```python
from build123d import *

# Parameters (mm, degrees)
SKETCH1_R           = 98.425
SKETCH1_R_2         = 8.89
BOSS_EXTRUDE1_DEPTH = 3.175


with BuildPart() as part:
    # Sketch1 → Boss-Extrude1 (new body)
    with BuildSketch(Plane(origin=(0, 0, 0), x_dir=(1, 0, 0), z_dir=(0, 1, 0))):
        Circle(SKETCH1_R)
        Circle(SKETCH1_R_2, mode=Mode.SUBTRACT)
        with BuildLine():
            Line((-5.5, 22.5), (-5.5, 67.5))
            ThreePointArc((-5.5, 67.5), (0, 73), (5.5, 67.5))
            Line((5.5, 67.5), (5.5, 22.5))
            ThreePointArc((5.5, 22.5), (0, 17), (-5.5, 22.5))
        make_face(mode=Mode.SUBTRACT)
    extrude(amount=BOSS_EXTRUDE1_DEPTH)


solid = part.part
```
Geometry: final body of the model. Coordinates: model frame, mm. A direction names the side the tool comes from. Coordinates: 2 decimals unless noted, no trailing zeros. Write each loop counter-clockwise with the first axis right and the second up, starting at its lowest first coordinate (ties: lowest second). Pieces come first, ordered by that corner, then holes. Notation, with made-up numbers: M -23,-19.75 L 29,-19.75 A9 cw 29,-4.75 Z; hole C 18,42.25 d6. An arc over 180 degrees is marked long. Use CSV: the item, a comma, the result in double quotes. Start each with the question number.
1. Mould query, pull axis Z, two halves, no side actions, for faces 3 (the face through (-1.93, 1.57, 8.68)), 4 (the face through (-1, 0, 20)), 5 (the face through (93.88, 1.57, -29.56)). Classes: pulls with the +Z half, pulls with the -Z half, needs draft (parallel to the pull), parting line crosses it, or undercut.
2. First-contact query: P1, Ø1.5, axis at y = 1, z = -68, coming from the +X side; P2, Ø1.5, axis at y = 0.5, z = 78, coming from the -X side; P3, Ø1.6, axis at y = 1, z = -38.5, coming from the +X side. Flat tips, straight axial feed; report the tip coordinate or a pass-through.
3. Cut plane A-A on x = 0. Return the cut outline in (y, z) (3 decimals).
4. Cut plane D-D on z = -25.5. Return the cut outline in (x, y) (3 decimals).
5. Cut plane C-C on y = 1.9. Return the cut outline in (x, z) (3 decimals), plus the area to 3 significant figures.
6. Reachability of faces 1 (the face through (-1, 3.175, 20)), 2 (the face through (0, 2, -73)) from +Z, -Z, +X, -X, +Y, -Y: full face, straight path, thin tool, end or side. Return the list, or none.
7. Ray query, probe 1 along Z at (x, y) = (0, 0.95) (3 decimals); probe 2 along X at (y, z) = (0.9, 0) (3 decimals); probe 3 along X at (y, z) = (0.8, 2.5). Return the intervals inside material, ascending.
8. Cut plane B-B on z = 0. Return the cut outline in (x, y) (3 decimals), plus the area to 3 significant figures.
Entries:
1,face 3,"undercut"
1,face 4,"needs draft"
1,face 5,"parting line crosses it"
2,P1,"x = 71.87"
2,P2,"x = -60.99"
2,P3,"x = 90.92"
3,outline,"M 0,-98.425 L 3.175,-98.425 L 3.175,-73 L 0,-73 Z; M 0,-17 L 3.175,-17 L 3.175,-8.89 L 0,-8.89 Z; M 0,8.89 L 3.175,8.89 L 3.175,98.425 L 0,98.425 Z"
4,outline,"M -95.064,0 L -5.5,0 L -5.5,3.175 L -95.064,3.175 Z; M 5.5,0 L 95.064,0 L 95.064,3.175 L 5.5,3.175 Z"
5,outline,"C 0,0 d196.85; hole C 0,0 d17.78; hole M -5.5,-67.5 A5.5 ccw 5.5,-67.5 L 5.5,-22.5 A5.5 ccw -5.5,-22.5 Z"
5,area,"29,600 mm²"
6,face 1,"+Z, -Z, +X, -X, +Y"
6,face 2,"+Y, -Y"
7,probe 1,"-98.425 to -73, -17 to -8.89, 8.89 to 98.425"
7,probe 2,"-98.425 to -8.89, 8.89 to 98.425"
7,probe 3,"-98.39 to -8.53, 8.53 to 98.39"
8,outline,"M -98.425,0 L -8.89,0 L -8.89,3.175 L -98.425,3.175 Z; M 8.89,0 L 98.425,0 L 98.425,3.175 L 8.89,3.175 Z"
8,area,"569 mm²"
